from build123d import *

# Parameters (mm, degrees)
SKETCH1_W           = 2.49
SKETCH1_H           = 5.21
SKETCH2_W           = 6.057828243
SKETCH2_H           = 1
BOSS_EXTRUDE2_DEPTH = 2.5
SKETCH4_W           = 0.5
SKETCH4_H           = 0.5
SKETCH4_W_2         = 0.535652732
SKETCH4_H_2         = 0.535652732
BOSS_EXTRUDE3_DEPTH = 20.3


with BuildPart() as part:
    # Sketch1 → Revolve3 (revolve)
    with BuildSketch(Plane.XY, mode=Mode.PRIVATE) as revolve3_sk:
        with Locations((1.245, -2.605)):
            Rectangle(SKETCH1_W, SKETCH1_H)
        with BuildLine():
            Line((0, 0), (2.49, 0))
            ThreePointArc((2.49, 0), (1.760695885, 1.760695885), (0, 2.49))
            Line((0, 2.49), (0, 0))
        make_face()
    revolve(revolve3_sk.sketch.rotate(Axis((0, 2.49, 0), (0, -1, 0)), 180), axis=Axis((0, 2.49, 0), (0, -1, 0)))

    # Sketch2 → Boss-Extrude2 (add, symmetric)
    with BuildSketch(Plane.XY):
        with Locations((-0.344367629, -5.71)):
            Rectangle(SKETCH2_W, SKETCH2_H)
    extrude(amount=BOSS_EXTRUDE2_DEPTH, both=True)

    # Sketch4 → Boss-Extrude3 (add)
    with BuildSketch(Plane.XZ.offset(6.21)):
        with Locations((-1.27, 0)):
            Rectangle(SKETCH4_W, SKETCH4_H)
        with Locations((1.27, 0)):
            Rectangle(SKETCH4_W_2, SKETCH4_H_2)
    extrude(amount=BOSS_EXTRUDE3_DEPTH)


solid = part.part
Verification items for the finished model (mm, model axes). A direction names the side the tool comes from. Give positions to 0.01 mm unless a question says otherwise; leave off trailing zeros. Order: outer loops, then holes, each group sorted by start corner. A loop starts at its lowest first (then second) coordinate and runs counter-clockwise, first axis right, second up. Notation, with made-up numbers: M 73.5,51.5 L 99.5,51.5 A16 cw 99.5,57.5 Z; hole C 47.5,62.5 d6. An arc over 180 degrees is marked long. Answer as a JSON object with one key per item and string values. Group by question number.
1) Depth check by flat-ended pin: pin 1 Ø3 at (x, y) = (1.5, -17) entering from +Z; pin 2 Ø3 at (x, z) = (-2.5, 1) entering from +Y; pin 3 Ø1.5 at (y, z) = (-20.5, 0) entering from -X. Enter the tip coordinate at first touch or a pass-through.
2) Cross-section at B-B (y = -22.5). Enter the section's corners in (x, z).
3) Cross-section at D-D (y = -4). Enter the section's corners in (x, z).
4) Cross-section at A-A (z = 0). Enter the section's corners in (x, y).
5) Scan lines: line 1 along X through (y, z) = (-19.5, -0.2); line 2 along Z through (x, y) = (-1.25, -8.25); line 3 along Y through (x, z) = (-2.25, -1.65). Record each from-to range of solid material in increasing order. Write a range as [from, to].
6) Mould release check, pull along X, two halves, no side actions. Record for faces 1 (the face through (-2.375, -2.569, -0.748)), 2 (the face through (0, -6, -2.5)), 3 (the face through (2.685, -6, 0)): released by +X, released by -X, zero draft, split by the parting line, or undercut.
7) Access from +Z, -Z, +X, -X, +Y, -Y to the whole of each face (thin tool, end or side, straight path). Record for faces 4 (the face through (-3.373, -6, 0)), 5 (the face through (-3, -5.21, 0)).
Result sheet:
{
 "1": {"pin 1": "stops at z = 0.27", "pin 2": "stops at y = 2.19", "pin 3": "stops at x = -1.52"},
 "2": {"outline": "M -1.52,-0.25 L -1.02,-0.25 L -1.02,0.25 L -1.52,0.25 Z; M 1,-0.27 L 1.54,-0.27 L 1.54,0.27 L 1,0.27 Z"},
 "3": {"outline": "C 0,0 d4.98"},
 "4": {"outline": "M -3.37,-6.21 L -1.52,-6.21 L -1.52,-26.51 L -1.02,-26.51 L -1.02,-6.21 L 1,-6.21 L 1,-26.51 L 1.54,-26.51 L 1.54,-6.21 L 2.68,-6.21 L 2.68,-5.21 L 2.49,-5.21 L 2.49,0 A2.49 ccw -2.49,0 L -2.49,-5.21 L -3.37,-5.21 Z"},
 "5": {"line 1": "x = [-1.52, -1.02], [1, 1.54]", "line 2": "z = [-0.25, 0.25]", "line 3": "y = [-6.21, -5.21]"},
 "6": {"face 1": "split by the parting line", "face 2": "zero draft", "face 3": "released by +X"},
 "7": {"face 4": "+Z, -Z, -X, +Y, -Y", "face 5": "+Y"}
}
